Design review of the part built by this model. Coordinates are the model's own, in mm. Face numbers are marked on the shaded views. Round coordinates to 2 decimals unless told otherwise and drop trailing zeros. Loops run counter-clockwise (first coordinate to the right, second up) from the corner with the lowest first, then second, coordinate; pieces in that order, holes last. Notation, with made-up numbers: (16.5, -31) -> (42.5, -31) arc R19 cw to (42.5, -19) -> close; hole circle Ø7 at (24, 1.5). An arc over 180 degrees is marked (long way). Write each question's results on one line, items separated by ' | '. Start each with the question number.
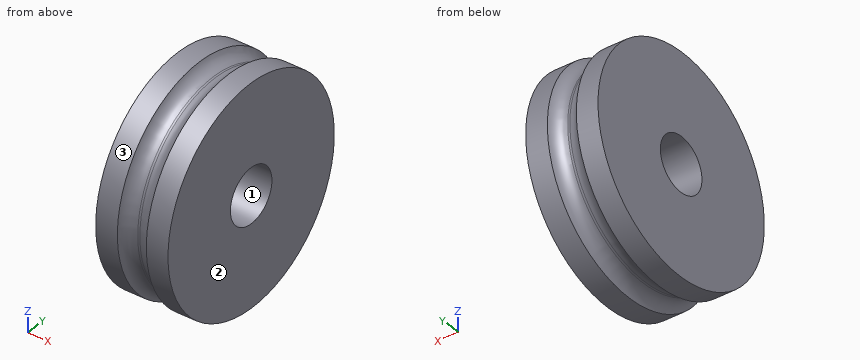
from build123d import *

# Parameters (mm, degrees)
FILLET1_R = 2.54


with BuildPart() as part:
    # Sketch1 → Revolve1 (revolve)
    with BuildSketch(Plane.XY, mode=Mode.PRIVATE) as revolve1_sk:
        Polygon((6.35, 4.7625), (-6.35, 4.7625), (-6.35, 19.05), (-2.54, 19.05), (-2.54, 17.4625), (2.54, 17.4625), (2.54, 19.05), (6.35, 19.05), align=None)
    revolve(revolve1_sk.sketch.rotate(Axis((-4.187009613, 0, 0), (1, 0, 0)), 90), axis=Axis((-4.187009613, 0, 0), (1, 0, 0)))

    # Fillet1
    # the kernel refuses this fillet: 2.54 mm, written as the material it adds along each edge
    with BuildSketch(Plane(origin=(-2.54, 0, 0), x_dir=(0, 0, 1), z_dir=(0, 1, 0))) as fillet1_piece_1:
        with BuildLine():
            CenterArc((20.0025, 2.35464302), FILLET1_R, 180, 67.975687163)
            Line((17.4625, 2.35464302), (17.4117, 2.35464302))
            Line((17.4117, 2.35464302), (17.4117, 0))
            Line((17.4117, 0), (17.4625, -0.0508))
            ThreePointArc((17.4625, -0.0508), (18.25625, -0.0508), (19.03095, -0.04709286))
            Line((19.03095, -0.04709286), (19.05, 0))
        make_face()
    revolve(axis=Axis((-2.54, 0, 0), (1, 0, 0)))
    with BuildSketch(Plane(origin=(2.54, 0, 0), x_dir=(0, 0, 1), z_dir=(0, 1, 0))) as fillet1_piece_2:
        with BuildLine():
            CenterArc((20.0025, -2.35464302), FILLET1_R, 112.024312837, 67.975687163)
            Line((19.05, 0), (19.03095, 0.04709286))
            ThreePointArc((19.03095, 0.04709286), (18.25625, 0.0508), (17.4625, 0.0508))
            Line((17.4625, 0.0508), (17.4117, 0))
            Line((17.4117, 0), (17.4117, -2.35464302))
            Line((17.4117, -2.35464302), (17.4625, -2.35464302))
        make_face()
    revolve(axis=Axis((2.54, 0, 0), (1, 0, 0)))


solid = part.part
1) Take a section at D-D (x = 1). Write out the cut boundary in (y, z) (1 decimal).
2) Take a section at A-A (y = 0). Write out the cut boundary in (x, z), plus the area to 3 significant figures.
3) To check wall thickness, follow line 1 (Y direction, x = -1.5, z = 0); line 2 (Y direction, x = -1, z = 0); line 3 (X direction, y = -8.5, z = -17). State the ranges of each line that lie inside material, in increasing order. Write a range as from..to.
4) Insertion check: pin 1 (3 mm diameter, centred on x = -0.5, y = 2, fed in from -Z); pin 2 (1 mm diameter, centred on x = 4.5, y = -9.5, fed in from +Z); pin 3 (2 mm diameter, centred on x = 3, z = 11.5, fed in from -Y). Each pin has a flat end and moves straight along its axis. Give the tip position at first contact, or say it passes through.
5) The part is to be moulded in two halves that separate along Y. For the marked faces 1, 2 and 3, say which applies: +Y half, -Y half, draft (parallel to the pull), parting line (faces both ways), or undercut.
Geometry check:
1) outline: circle Ø35.2 at (0, 0); hole circle Ø9.5 at (0, 0)
2) outline: (-6.35, -19.05) -> (-2.54, -19.05) arc R2.54 cw to (-0.19, -17.46) -> (0.19, -17.46) arc R2.54 cw to (2.54, -19.05) -> (6.35, -19.05) -> (6.35, -4.76) -> (-6.35, -4.76) -> close; (-6.35, 4.76) -> (6.35, 4.76) -> (6.35, 19.05) -> (2.54, 19.05) arc R2.54 cw to (0.19, 17.46) -> (-0.19, 17.46) arc R2.54 cw to (-2.54, 19.05) -> (-6.35, 19.05) -> close | area: 351 mm^2
3) line 1: y = -17.83..-4.76, 4.76..17.83 | line 2: y = -17.6..-4.76, 4.76..17.6 | line 3: x = -6.35..-2.52, 2.52..6.35
4) pin 1: stops at z = -18.12 | pin 2: stops at z = 16.79 | pin 3: stops at y = -15.9
5) face 1: undercut | face 2: draft | face 3: parting line
